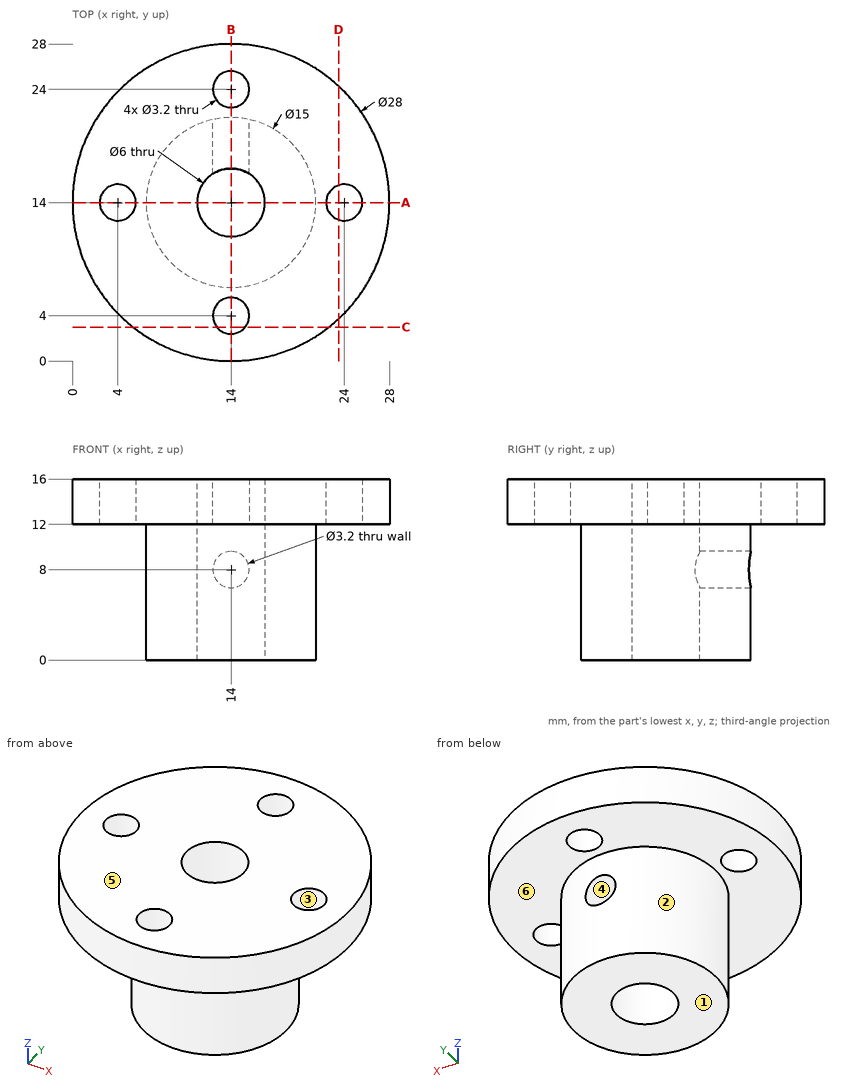
The drawing under review shows one solid part. Ordinate dimensions are in mm from its lowest x, y, z. A direction names the side the tool comes from. Give positions to 0.01 mm unless a question says otherwise; leave off trailing zeros. Write each loop counter-clockwise with the first axis right and the second up, starting at its lowest first coordinate (ties: lowest second). Pieces come first, ordered by that corner, then holes. Notation, with made-up numbers: (4, -37.5) - (58, -37.5) arc R26 ccw to (58, -21.5) - close; hole circle Ø8 at (50.5, -20). An arc over 180 degrees is marked (long way). Answer in a Markdown table with one row per item. Add a question column.
1. Insertion check: P1, Ø1.5, axis at x = 5.5, z = 10, coming from the -Y side; P2, Ø4, axis at y = 9.5, z = 12.5, coming from the -X side (3 decimals); P3, Ø4, axis at x = 25, z = 12.5, coming from the +Y side; P4, Ø4, axis at y = 15.5, z = 3, coming from the +X side. Each pin has a flat end and moves straight along its axis. Give the tip position at first contact, or say it passes through.
2. We need section B-B on x = 14. Write out the cut boundary in (y, z), then the cut area to 3 significant figures.
3. Tool access review of the marked faces 4, 5 and 6: name each direction out of +Z, -Z, +X, -X, +Y, -Y from which nothing blocks a thin tool from reaching the whole face with its end or side.
4. We need section A-A on y = 14. Write out the cut boundary in (x, z), then the cut area to 3 significant figures.
5. We need section D-D on x = 23.5. Write out the cut boundary in (y, z).
6. We need section C-C on y = 3. Write out the cut boundary in (x, z).
7. Wall thickness on line 1 along Y through (x, z) = (14, 12.75); line 2 along Z through (x, y) = (8, 19.25); line 3 along X through (y, z) = (17.8, 8): over which ranges is each line inside the solid? List them lowest first. Write a range as [from, to].
8. Draft analysis for pull direction Y (two halves, no side actions). For the marked faces 1, 2 and 3, state which applies: +Y half, -Y half, draft (parallel to the pull), parting line (faces both ways), or undercut.
Ans:
| question | item | result |
|---|---|---|
| 1 | P1 | passes through |
| 1 | P2 | stops at x = 0.225 |
| 1 | P3 | stops at y = 24.72 |
| 1 | P4 | stops at x = 21.5 |
| 2 | outline | (0, 12) - (2.4, 12) - (2.4, 16) - (0, 16) - close; (5.6, 12) - (6.5, 12) - (6.5, 0) - (11, 0) - (11, 16) - (5.6, 16) - close; (17, 0) - (21.5, 0) - (21.5, 6.4) - (17, 6.4) - close; (17, 9.6) - (21.5, 9.6) - (21.5, 12) - (22.4, 12) - (22.4, 16) - (17, 16) - close; (25.6, 12) - (28, 12) - (28, 16) - (25.6, 16) - close |
| 2 | area | 156 mm^2 |
| 3 | face 4 | +Y |
| 3 | face 5 | +Z, +X, -X, +Y, -Y |
| 3 | face 6 | -Z |
| 4 | outline | (0, 12) - (2.4, 12) - (2.4, 16) - (0, 16) - close; (5.6, 12) - (6.5, 12) - (6.5, 0) - (11, 0) - (11, 16) - (5.6, 16) - close; (17, 0) - (21.5, 0) - (21.5, 12) - (22.4, 12) - (22.4, 16) - (17, 16) - close; (25.6, 12) - (28, 12) - (28, 16) - (25.6, 16) - close |
| 4 | area | 170 mm^2 |
| 5 | outline | (3.72, 12) - (12.48, 12) - (12.48, 16) - (3.72, 16) - close; (15.52, 12) - (24.28, 12) - (24.28, 16) - (15.52, 16) - close |
| 6 | outline | (5.34, 12) - (12.75, 12) - (12.75, 16) - (5.34, 16) - close; (15.25, 12) - (22.66, 12) - (22.66, 16) - (15.25, 16) - close |
| 7 | line 1 | y = [0, 2.4], [5.6, 11], [17, 22.4], [25.6, 28] |
| 7 | line 2 | z = [12, 16] |
| 7 | line 3 | x = [7.53, 12.4], [15.6, 20.47] |
| 8 | face 1 | draft |
| 8 | face 2 | parting line |
| 8 | face 3 | undercut |
